Design review of the part built by this model. Coordinates are the model's own, in mm. A direction names the side the tool comes from. Coordinates: 2 decimals unless noted, no trailing zeros. Loops run counter-clockwise (first coordinate to the right, second up) from the corner with the lowest first, then second, coordinate; pieces in that order, holes last.
Q1. Add section B-B on y = 6.5. Give the boundary of the cut face in (x, z).
Q2. Add section A-A on z = 13.5. Give the boundary of the cut face in (x, y).
Q3. Wall thickness on probe 1 along X at (y, z) = (0, 8); probe 2 along X at (y, z) = (1, 7.5); probe 3 along X at (y, z) = (0, 24): over which ranges is each line inside the solid? List them lowest first.
Q4. Add section C-C on z = 28.5. Give the boundary of the cut face in (x, y), and give its area (3 significant figures).
Q5. For P1, Ø8, axis at x = -41, y = -0.5, coming from the +Z side; P2, Ø12, axis at x = 24, z = 6, coming from the -Y side; P3, Ø1.5, axis at x = -17, z = 5, coming from the +Y side; P4, Ø11, axis at x = -11, z = 30.5, coming from the +Y side, all flat-tipped, find the tip position at first contact; note any pin that passes through.
Q6. Add section D-D on x = -13. Give the boundary of the cut face in (y, z), and give its area (3 significant figures).
Q7. Draft analysis for pull direction Y (two halves, no side actions). For faces 1 (the face through (-27, 13, 35)), 2 (the face through (-41, 0, 25)), 3 (the face through (47.97, -0.73, 7.4)), state which applies: released by +Y, released by -Y, zero draft, split by the parting line, or undercut.
Q8. Machinability: for faces 4 (the face through (-13, -5, 30)), 5 (the face through (0, 0, 0)), which of the approach directions +Z, -Z, +X, -X, +Y, -Y give a long, thin tool a straight path to every point of the face, cutting with its end or side? Answer none if there is none.
```python
from build123d import *

# Parameters (mm, degrees)
F1_DEPTH = 15
F3_DEPTH = 20
F4_R     = 10
F5_DEPTH = 60.8
F7_DEPTH = 10
F9_DEPTH = 33.1


with BuildPart() as f1:
    # F0 (on Top) → F1 (new body)
    with BuildSketch(Plane.XY):
        with BuildLine():
            Line((-27.8139331382, 19.9841398605), (-26.2326190666, 19.9845893727))
            ThreePointArc((-26.2326190666, 19.9845893727), (-27.0232805468, 19.9999991919), (-27.8139331382, 19.9841398605))
        make_face()
        with BuildLine():
            Line((27.9767194532, 19.9999991919), (-26.2326190666, 19.9845893727))
            Line((-26.2326190666, 19.9845893727), (-27.8139331382, 19.9841398605))
            ThreePointArc((-27.8139331382, 19.9841398605), (-47.0135984526, -0.399819681), (-27.0144510727, -19.9999997529))
            Line((-27.0144510727, -19.9999997529), (27.397513264, -19.9914457192))
            ThreePointArc((27.397513264, -19.9914457192), (47.9803074375, -0.2896346714), (27.9767194532, 19.9999991919))
        make_face()
    extrude(amount=F1_DEPTH)

    # F2 (on face) → F3 (join)
    with BuildSketch(Plane.XY.offset(15)):
        with BuildLine():
            ThreePointArc((-27.0144510727, -19.9999997529), (-12.8743480331, -14.1410239467), (-7.0175952464, 0))
            ThreePointArc((-7.0175952464, 0), (-12.600599658, 13.8618266546), (-26.2326190666, 19.9845893727))
            ThreePointArc((-26.2326190666, 19.9845893727), (-47.0137730139, 0.3909919326), (-27.0144510727, -19.9999997529))
        make_face()
    extrude(amount=F3_DEPTH)

    # F4 (on face) → F5 (cut)
    with BuildSketch(Plane.XY.offset(35)):
        with Locations((-27.0175952464, 0)):
            Circle(F4_R)
    extrude(amount=-F5_DEPTH, mode=Mode.SUBTRACT)

    # F6 (on face) → F7 (cut)
    with BuildSketch(Plane.XY.offset(35)):
        with BuildLine():
            Line((-46.3825119775, 5), (-53.2571481913, 5))
            Line((-53.2571481913, 5), (-53.2571481913, -5))
            Line((-53.2571481913, -5), (-46.3825119775, -5))
            ThreePointArc((-46.3825119775, -5), (-47.0175952464, 0), (-46.3825119775, 5))
        make_face()
        with BuildLine():
            Line((6.7428518087, 5), (-7.6526785154, 5))
            ThreePointArc((-7.6526785154, 5), (-7.1770013211, 2.5200858497), (-7.0175952464, 0))
            ThreePointArc((-7.0175952464, 0), (-7.1770013211, -2.5200858497), (-7.6526785154, -5))
            Line((-7.6526785154, -5), (6.7428518087, -5))
            Line((6.7428518087, -5), (6.7428518087, 5))
        make_face()
        with BuildLine():
            Line((-35.6778492843, 5), (-46.3825119775, 5))
            ThreePointArc((-46.3825119775, 5), (-47.0175952464, 0), (-46.3825119775, -5))
            Line((-46.3825119775, -5), (-35.6778492843, -5))
            ThreePointArc((-35.6778492843, -5), (-37.0175952464, 0), (-35.6778492843, 5))
        make_face()
        with BuildLine():
            Line((-18.3573412086, 5), (-35.6778492843, 5))
            ThreePointArc((-35.6778492843, 5), (-37.0175952464, 0), (-35.6778492843, -5))
            Line((-35.6778492843, -5), (-18.3573412086, -5))
            ThreePointArc((-18.3573412086, -5), (-17.3583369835, -2.588190451), (-17.0175952464, 0))
            ThreePointArc((-17.0175952464, 0), (-17.3583369835, 2.588190451), (-18.3573412086, 5))
        make_face()
        with BuildLine():
            ThreePointArc((-7.0175952464, 0), (-7.1770013211, 2.5200858497), (-7.6526785154, 5))
            Line((-7.6526785154, 5), (-18.3573412086, 5))
            ThreePointArc((-18.3573412086, 5), (-17.3583369835, 2.588190451), (-17.0175952464, 0))
            ThreePointArc((-17.0175952464, 0), (-17.3583369835, -2.588190451), (-18.3573412086, -5))
            Line((-18.3573412086, -5), (-7.6526785154, -5))
            ThreePointArc((-7.6526785154, -5), (-7.1770013211, -2.5200858497), (-7.0175952464, 0))
        make_face()
    extrude(amount=-F7_DEPTH, mode=Mode.SUBTRACT)

    # F8 (on face) → F9 (cut)
    with BuildSketch(Plane.XY.offset(15)):
        with BuildLine():
            Line((28.2606767434, -7.4948358688), (27.7091998301, -7.4950222861))
            ThreePointArc((27.7091998301, -7.4950222861), (27.9849400007, -7.4999995715), (28.2606767434, -7.4948358688))
        make_face()
        with BuildLine():
            Line((12.9849400007, -7.4999995715), (27.7091998301, -7.4950222861))
            Line((27.7091998301, -7.4950222861), (28.2606767434, -7.4948358688))
            ThreePointArc((28.2606767434, -7.4948358688), (35.4811133003, 0.1391766201), (27.9823714109, 7.5))
            Line((27.9823714109, 7.5), (13.0139985431, 7.4999334552))
            ThreePointArc((13.0139985431, 7.4999334552), (12.9823714109, 7.4999999999), (12.9507442793, 7.499933174))
            ThreePointArc((12.9507442793, 7.499933174), (5.4824242428, -0.017097893), (12.9849400007, -7.4999995715))
        make_face()
    extrude(amount=-F9_DEPTH, mode=Mode.SUBTRACT)


solid = f1.part
```
Entries:
1. outline: (-45.93, 0) - (-34.62, 0) - (-34.62, 35) - (-45.93, 35) - close; (-19.42, 0) - (9.24, 0) - (9.24, 15) - (-8.1, 15) - (-8.1, 35) - (-19.42, 35) - close; (31.72, 0) - (46.9, 0) - (46.9, 15) - (31.72, 15) - close
2. outline: (-27.01, -20) - (27.4, -19.99) arc R20 ccw (long way) to (27.98, 20) - (-26.23, 19.98) arc R20 ccw (long way) to start; hole circle Ø20 at (-27.02, 0); hole (12.95, 7.5) arc R7.5 ccw to (12.98, -7.5) - (27.71, -7.5) arc R7.5 ccw (long way) to (27.98, 7.5) - (13.01, 7.5) arc R7.5 ccw to start
3. probe 1: x = -47.02 to -37.02, -17.02 to 5.48, 35.48 to 47.98
3. probe 2: x = -46.99 to -36.97, -17.07 to 5.55, 35.42 to 47.96
3. probe 3: x = -47.02 to -37.02, -17.02 to -7.02
4. outline: (-46.38, -5) arc R20 ccw to (-7.65, -5) - (-18.36, -5) arc R10 cw to (-35.68, -5) - close; (-46.38, 5) - (-35.68, 5) arc R10 cw to (-18.36, 5) - (-7.65, 5) arc R20 ccw to start
4. area: 738 mm2
5. P1: stops at z = 25
5. P2: stops at y = -20
5. P3: stops at y = 19.99
5. P4: stops at y = 17.01
6. outline: (-20, 0) - (19.99, 0) - (19.99, 15) - (14.27, 15) - (14.27, 35) - (5, 35) - (5, 25) - (-5, 25) - (-5, 35) - (-14.27, 35) - (-14.27, 15) - (-20, 15) - close
6. area: 1,070 mm2
7. face 1: zero draft
7. face 2: undercut
7. face 3: split by the parting line
8. face 4: +Z, +X, -X
8. face 5: -Z, +X, -X, +Y, -Y
